```python
from build123d import *
from build123d.topology import SkipClean

# Parameters (mm, degrees)
SKETCH_1_R          = 6
EXTRUDE_1_DEPTH     = 9
CUT_EXTRUDE_1_DEPTH = 13.369316877
SKETCH_3_R          = 6
EXTRUDE_2_DEPTH     = 3
SKETCH_4_R          = 1.5
CUT_EXTRUDE_2_DEPTH = 3
EXTRUDE_3_DEPTH     = 2
SKETCH_7_R          = 7
EXTRUDE_4_DEPTH     = 3
SKETCH_8_R          = 5.8
EXTRUDE_5_DEPTH     = 2.2
SKETCH_9_R          = 1.3
CUT_EXTRUDE_3_DEPTH = 6
CHAMFER_1_SIZE      = 1
SKETCH_10_W         = 6
SKETCH_10_H         = 6
EXTRUDE_6_DEPTH     = 6
SKETCH_11_R         = 1.25
CUT_EXTRUDE_4_DEPTH = 8


with BuildPart() as part:
    # Эскиз1 → Бобышка-Вытянуть1 (new body)
    with BuildSketch(Plane(origin=(0, 0, 0), x_dir=(1, 0, 0), z_dir=(0, 1, 0))):
        with Locations(Location((0, 0, 0), (0, 0, 270))):
            Circle(SKETCH_1_R)
    extrude(amount=EXTRUDE_1_DEPTH)

    # Эскиз2 → Вырез-Вытянуть1 (cut, through all)
    with BuildSketch(Plane(origin=(0, 9, 0), x_dir=(1, 0, 0), z_dir=(0, 1, 0))):
        with BuildLine():
            Line((-1.28, 1.404136745), (-1.28, -1.404136745))
            ThreePointArc((-1.28, -1.404136745), (1.9, 0), (-1.28, 1.404136745))
        make_face()
    extrude(amount=-CUT_EXTRUDE_1_DEPTH, mode=Mode.SUBTRACT)

    # Эскиз3 → Бобышка-Вытянуть2 (add)
    with BuildSketch(Plane(origin=(0, 9, 0), x_dir=(1, 0, 0), z_dir=(0, 1, 0))):
        with Locations(Location((0, 0, 0), (0, 0, 270))):
            Circle(SKETCH_3_R)
    extrude(amount=EXTRUDE_2_DEPTH)

    # Эскиз4 → Вырез-Вытянуть2 (cut)
    with BuildSketch(Plane(origin=(0, 12, 0), x_dir=(1, 0, 0), z_dir=(0, 1, 0))):
        with Locations(Location((0, 0, 0), (0, 0, 270))):
            Circle(SKETCH_4_R)
    extrude(amount=-CUT_EXTRUDE_2_DEPTH, mode=Mode.SUBTRACT)

    # Эскиз5 → Бобышка-Вытянуть3 (add)
    with SkipClean():  # the faces are left unmerged after this step: merging them gives an invalid solid
        with BuildSketch(Plane(origin=(0, 12, 0), x_dir=(1, 0, 0), z_dir=(0, 1, 0))):
            with BuildLine():
                Line((5.454356057, 2.5), (-5.454356057, 2.5))
                ThreePointArc((-5.454356057, 2.5), (0, 6), (5.454356057, 2.5))
            make_face()
            with BuildLine():
                Line((5.454356057, -2.5), (-5.454356057, -2.5))
                ThreePointArc((-5.454356057, -2.5), (0, -6), (5.454356057, -2.5))
            make_face()
        extrude(amount=EXTRUDE_3_DEPTH)

    # Эскиз7 → Бобышка-Вытянуть4 (add)
    with BuildSketch(Plane(origin=(0, 14, 0), x_dir=(1, 0, 0), z_dir=(0, 1, 0))):
        with Locations(Location((0, 0, 0), (0, 0, 270))):
            Circle(SKETCH_7_R)
    extrude(amount=EXTRUDE_4_DEPTH)

    # Эскиз8 → Бобышка-Вытянуть5 (add)
    with BuildSketch(Plane(origin=(0, 17, 0), x_dir=(1, 0, 0), z_dir=(0, 1, 0))):
        with Locations(Location((0, 0, 0), (0, 0, 270))):
            Circle(SKETCH_8_R)
    extrude(amount=EXTRUDE_5_DEPTH)

    # Эскиз9 → Вырез-Вытянуть3 (cut)
    with BuildSketch(Plane(origin=(0, 19.2, 0), x_dir=(1, 0, 0), z_dir=(0, 1, 0))):
        with Locations(Location((0, 0, 0), (0, 0, 270))):
            Circle(SKETCH_9_R)
    extrude(amount=-CUT_EXTRUDE_3_DEPTH, mode=Mode.SUBTRACT)

    # Фаска1
    # the kernel refuses this chamfer: 1 mm, written as the material it adds along each edge
    with BuildSketch(Plane(origin=(0, 14, 0), x_dir=(-0.9999996815285755, 0, -0.0007980869299166744), z_dir=(-0.0007980869299166744, 0, 0.9999996815285755))) as chamfer_1_piece_1_section:
        Polygon((6 + CHAMFER_1_SIZE, 0), (6, CHAMFER_1_SIZE), (6, 0), align=None)
    chamfer_1_piece_1 = revolve(axis=Axis((0, 14, 0), (0, -1, 0)), revolution_arc=179.908545965, mode=Mode.PRIVATE)
    chamfer_1_piece_1 = chamfer_1_piece_1 & Plane(origin=(0, 13.500057011, 0), x_dir=(0, 0, 1), z_dir=(0, -1, 0)) * Cylinder(7, 28, mode=Mode.PRIVATE)
    chamfer_1_piece_1 = split(chamfer_1_piece_1, bisect_by=Plane(origin=(0, 13.500057011, -2.5), z_dir=(0, 0, -1)), keep=Keep.TOP, mode=Mode.PRIVATE)
    add(chamfer_1_piece_1)
    with BuildSketch(Plane(origin=(0, 14, 0), x_dir=(-0.9999996815285755, 0, 0.0007980869299168965), z_dir=(-0.0007980869299168965, 0, -0.9999996815285755))) as chamfer_1_piece_2_section:
        Polygon((6 + CHAMFER_1_SIZE, 0), (6, -CHAMFER_1_SIZE), (6, 0), align=None)
    chamfer_1_piece_2 = revolve(axis=Axis((0, 14, 0), (0, 1, 0)), revolution_arc=179.908545965, mode=Mode.PRIVATE)
    chamfer_1_piece_2 = chamfer_1_piece_2 & Plane(origin=(0, 13.500057011, 0), x_dir=(0, 0, 1), z_dir=(0, -1, 0)) * Cylinder(7, 28, mode=Mode.PRIVATE)
    chamfer_1_piece_2 = split(chamfer_1_piece_2, bisect_by=Plane(origin=(0, 13.500057011, 2.5), z_dir=(0, 0, 1)), keep=Keep.TOP, mode=Mode.PRIVATE)
    add(chamfer_1_piece_2)
    # the kernel refuses this chamfer: 1 mm, written as the material it takes off along each edge
    with BuildSketch(Plane(origin=(0, 0, 0), x_dir=(0, 0, 1), z_dir=(-1, 0, 0))) as chamfer_1_2_piece_1:
        Polygon((6 - CHAMFER_1_SIZE, 0), (6, CHAMFER_1_SIZE), (6, 0), align=None)
    revolve(axis=Axis((0, 0, 0), (0, 1, 0)), mode=Mode.SUBTRACT)

    # Эскиз10 → Бобышка-Вытянуть6 (add)
    with BuildSketch(Plane(origin=(0, 19.2, 0), x_dir=(1, 0, 0), z_dir=(0, 1, 0))):
        Rectangle(SKETCH_10_W, SKETCH_10_H)
    extrude(amount=EXTRUDE_6_DEPTH)

    # Эскиз11 → Вырез-Вытянуть4 (cut)
    with BuildSketch(Plane(origin=(0, 25.2, 0), x_dir=(1, 0, 0), z_dir=(0, 1, 0))):
        with Locations(Location((0, 0, 0), (0, 0, 270))):
            Circle(SKETCH_11_R)
    extrude(amount=-CUT_EXTRUDE_4_DEPTH, mode=Mode.SUBTRACT)


solid = part.part
```
Work out the finished part from the listing and answer in its coordinate system (mm). A direction names the side the tool comes from. Give positions to 0.01 mm unless a question says otherwise; leave off trailing zeros. Loops run counter-clockwise (first coordinate to the right, second up) from the corner with the lowest first, then second, coordinate; pieces in that order, holes last. Notation, with made-up numbers: (-11, 11) - (9, 11) arc R27 ccw to (9, 38) - close; hole circle Ø1 at (-33, 82). An arc over 180 degrees is marked (long way). Use CSV: the item, a comma, the result in double quotes. Start each with the question number.
(1) Find section D-D, the plane y = 5.25. Determine the outline of the cut face in (x, z), plus the area to 3 significant figures.
(2) Find section A-A, the plane z = 0. Count the separate pieces of the cut face and the enclosed holes in it, plus the area to 3 significant figures.
(3) Each of these flat-tipped pins is pushed along its axis until it touches: pin 1 (2 mm diameter, centred on y = 4, z = 0.5, fed in from +X); pin 2 (6.5 mm diameter, centred on x = 1, y = 21.5, fed in from -Z); pin 3 (3 mm diameter, centred on x = -0.5, z = -0.5, fed in from -Y); pin 4 (3 mm diameter, centred on x = 0.5, y = 23, fed in from +Z). Where does it stop, or does it pass through?
(4) Find section C-C, the plane y = 14.75. Determine the outline of the cut face in (x, z), plus the area to 3 significant figures.
(5) A tool of negligible diameter and unlimited length cuts with its end or side. For faces 4 (the face through (1.61, 9, 0.41)), 5 (the face through (0, 22, -3)), 6 (the face through (2, 14, 0)), from which of +Z, -Z, +X, -X, +Y, -Y can it reach the whole face along a straight path? Write none if from no direction.
(6) Find section B-B, the plane y = 10. Determine the outline of the cut face in (x, z), plus the area to 3 significant figures.
(7) Find the intervals of material crossed by L1, parallel to Y at x = 4.25, z = 0.5; L2, parallel to Z at x = 0, y = 10; L3, parallel to Y at x = -2, z = -2.25, in increasing order.
(8) Determine the mould class of faces 1 (the face through (-1.22, 22.24, -0.27)), 2 (the face through (1, 25.2, -1)), 3 (the face through (-0.1, 13.2, 6.2)) for opening direction X: released by +X, released by -X, zero draft, split by the parting line, or undercut.
Results found:
1,outline,"circle Ø12 at (0, 0); hole (-1.28, -1.4) arc R1.9 ccw (long way) to (-1.28, 1.4) - close"
1,area,"103 mm^2"
2,separate pieces,"4"
2,enclosed holes,"0"
2,area,"180 mm^2"
3,pin 1,"x = 6"
3,pin 2,"z = -5.8"
3,pin 3,"y = 0"
3,pin 4,"z = 3"
4,outline,"circle Ø14 at (0, 0); hole circle Ø2.6 at (0, 0)"
4,area,"149 mm^2"
5,face 4,"-Y"
5,face 5,"-Z, +X, -X, +Y"
5,face 6,"+X, -X"
6,outline,"circle Ø12 at (0, 0); hole circle Ø3 at (0, 0)"
6,area,"106 mm^2"
7,L1,"0 to 12, 14 to 19.2"
7,L2,"-6 to -1.5, 1.5 to 6"
7,L3,"0 to 12, 14 to 25.2"
8,face 1,"undercut"
8,face 2,"zero draft"
8,face 3,"split by the parting line"
